from build123d import *

# Parameters (mm, degrees)
SKETCH1_W           = 1530
SKETCH1_H           = 230
BOSS_EXTRUDE3_DEPTH = 30
SKETCH9_R           = 27.5
CUT_EXTRUDE1_DEPTH  = 31.0000001
SKETCH10_W          = 1530
SKETCH10_H          = 980
BOSS_EXTRUDE4_DEPTH = 30
SKETCH11_W          = 980
SKETCH11_H          = 760
BOSS_EXTRUDE5_DEPTH = 30
SKETCH12_W          = 920
SKETCH12_H          = 30
BOSS_EXTRUDE6_DEPTH = 1530
SKETCH13_W          = 20
SKETCH13_H          = 200
BOSS_EXTRUDE7_DEPTH = 1530
SKETCH14_R          = 27.5
SKETCH14_R_2        = 40
CUT_EXTRUDE3_DEPTH  = 500
BOSS_EXTRUDE8_START = 500
SKETCH17_W          = 110
SKETCH17_H          = 24.94
BOSS_EXTRUDE8_DEPTH = 300


with BuildPart() as part:
    # Sketch1 → Boss-Extrude3 (new body)
    with BuildSketch(Plane.XY):
        with BuildLine():
            Line((765, 500), (-235, 500))
            add(Edge.make_bspline(
                [(-235, 500), (-580.943747407, 493.32484482), (-765, 200)],
                knots=[0, 0, 0, 1, 1, 1], degree=2))
            Line((-765, 200), (-765, 0))
            Line((-765, 0), (765, 0))
            Line((765, 0), (765, 500))
        make_face()
        with Locations((0, -115)):
            Rectangle(SKETCH1_W, SKETCH1_H)
    boss_extrude3 = extrude(amount=BOSS_EXTRUDE3_DEPTH)

    # Sketch9 → Cut-Extrude1 (cut, through all)
    with BuildSketch(Plane.XY.offset(30)):
        with Locations((-510, -130)):
            Circle(SKETCH9_R)
        with Locations((510, -130)):
            Circle(SKETCH9_R)
    cut_extrude1 = extrude(amount=-CUT_EXTRUDE1_DEPTH, mode=Mode.SUBTRACT)

    # Sketch10 → Boss-Extrude4 (add)
    with BuildSketch(Plane.XZ.offset(230)):
        with Locations((0, -460)):
            Rectangle(SKETCH10_W, SKETCH10_H)
    extrude(amount=BOSS_EXTRUDE4_DEPTH)

    # Sketch11 → Boss-Extrude5 (add)
    with BuildSketch(Plane(origin=(765, 0, 0), x_dir=(0, 0, -1), z_dir=(1, 0, 0))):
        with Locations((460, 120)):
            Rectangle(SKETCH11_W, SKETCH11_H)
    boss_extrude5 = extrude(amount=BOSS_EXTRUDE5_DEPTH)

    # Mirror3: Boss-Extrude3, Cut-Extrude1, Boss-Extrude5 across plane
    add(boss_extrude3.mirror(Plane.XY.offset(-460)))
    add(cut_extrude1.mirror(Plane.XY.offset(-460)), mode=Mode.SUBTRACT)
    add(boss_extrude5.mirror(Plane.XY.offset(-460)))

    # Sketch12 → Boss-Extrude6 (add)
    with BuildSketch(Plane.ZY.offset(-765)):
        with Locations((-460, -15)):
            Rectangle(SKETCH12_W, SKETCH12_H)
    extrude(amount=BOSS_EXTRUDE6_DEPTH)

    # Sketch13 → Boss-Extrude7 (add)
    with BuildSketch(Plane.ZY.offset(765)):
        with Locations((-670, -130)):
            Rectangle(SKETCH13_W, SKETCH13_H)
        with Locations((-250, -130)):
            Rectangle(SKETCH13_W, SKETCH13_H)
    extrude(amount=-BOSS_EXTRUDE7_DEPTH)

    # Sketch14 → Cut-Extrude3 (cut)
    with BuildSketch(Plane.XY.offset(-240)):
        with Locations((-510, -130)):
            Circle(SKETCH14_R)
        with Locations((0, -130)):
            Circle(SKETCH14_R_2)
        with Locations((510, -130)):
            Circle(SKETCH14_R)
    extrude(amount=-CUT_EXTRUDE3_DEPTH, mode=Mode.SUBTRACT)

    # Sketch17 → Boss-Extrude8 (add)
    with BuildSketch(Plane.ZY.offset(-765).offset(BOSS_EXTRUDE8_START)):
        with Locations((-460, -217.53)):
            Rectangle(SKETCH17_W, SKETCH17_H)
    extrude(amount=BOSS_EXTRUDE8_DEPTH)


solid = part.part
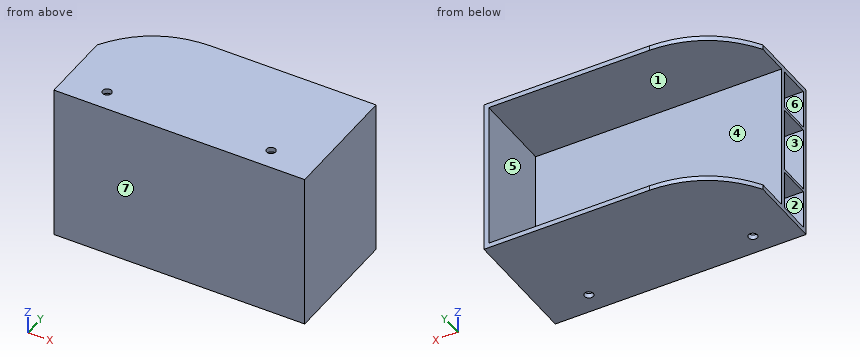
The listing builds one solid part. Answer for the finished solid, in the listing's coordinates (mm). Face numbers are marked on the shaded views. A direction names the side the tool comes from. Give positions to 0.01 mm unless a question says otherwise; leave off trailing zeros. Write each loop counter-clockwise with the first axis right and the second up, starting at its lowest first coordinate (ties: lowest second). Pieces come first, ordered by that corner, then holes. Notation, with made-up numbers: (49.25, 65.25) -> (63.25, 65.25) arc R13 ccw to (63.25, 90.25) -> close; hole circle Ø7 at (0.5, 38.5). An arc over 180 degrees is marked (long way). Use a Markdown table: item, result.
(1) For the marked faces 5, 6 and 7, determine the directions among +Z, -Z, +X, -X, +Y, -Y from which every point of the face is accessible in a straight line to the end or side of a thin tool.
Return value:
| item | result |
|---|---|
| face 5 | -X, +Y |
| face 6 | -X |
| face 7 | +Z, -Z, +X, -X, -Y |
(2) Find the intervals of material crossed by probe 1 along Z at (x, y) = (713, -57); probe 2 along X at (y, z) = (-130, -943.75); probe 3 along Z at (x, y) = (517, 206.5), in increasing order. Write a range as from..to.
Return value:
| item | result |
|---|---|
| probe 1 | -950..-920, -680..-660, -260..-240, 0..30 |
| probe 2 | -765..-537.5, -482.5..482.5, 537.5..795 |
| probe 3 | -950..-920, 0..30 |
(3) Flat-ended cylindrical pins translate along their axes: P1, Ø4, axis at y = 204.5, z = -813.5, coming from the -X side; P2, Ø3, axis at x = 65.5, z = -377.5, coming from the +Y side. Find the tip coordinate at first contact, or state that the pin passes through.
Return value:
| item | result |
|---|---|
| P1 | x = 765 |
| P2 | y = 0 |
(4) Section C-C, the plane y = -130 is taken. Give the number of separate pieces and of enclosed holes in the cut face, then the cut area to 3 significant figures.
Return value:
| item | result |
|---|---|
| separate pieces | 11 |
| enclosed holes | 0 |
| area | 168,000 mm2 |
(5) Section A-A, the plane x = 210.5 is taken. Determine the outline of the cut face in (y, z).
Return value:
| item | result |
|---|---|
| outline | (-260, -950) -> (500, -950) -> (500, -920) -> (0, -920) -> (0, 0) -> (500, 0) -> (500, 30) -> (-260, 30) -> close; hole (-230, -920) -> (-30, -920) -> (-30, -680) -> (-230, -680) -> close; hole (-230, -660) -> (-30, -660) -> (-30, -260) -> (-230, -260) -> (-230, -405) -> (-205.06, -405) -> (-205.06, -515) -> (-230, -515) -> close; hole (-230, -240) -> (-30, -240) -> (-30, 0) -> (-230, 0) -> close |
(6) Section D-D, the plane y = 82 is taken. Determine the outline of the cut face in (x, z).
Return value:
| item | result |
|---|---|
| outline | (-765, -950) -> (795, -950) -> (795, 30) -> (-765, 30) -> (-765, 0) -> (765, 0) -> (765, -920) -> (-765, -920) -> close |
(7) Section B-B, the plane z = -218 is taken. Determine the outline of the cut face in (x, y), then the cut area to 3 significant figures.
Return value:
| item | result |
|---|---|
| outline | (-765, -260) -> (795, -260) -> (795, 500) -> (765, 500) -> (765, 0) -> (-765, 0) -> (-765, -30) -> (765, -30) -> (765, -230) -> (-765, -230) -> close |
| area | 115,000 mm2 |
(8) Determine the mould class of the marked faces 1, 2, 3 and 4 for opening direction Y: released by +Y, released by -Y, zero draft, split by the parting line, or undercut.
Return value:
| item | result |
|---|---|
| face 1 | zero draft |
| face 2 | undercut |
| face 3 | undercut |
| face 4 | released by +Y |
